Drawing for the job (mm, zero at the part's lowest x, y, z). A direction names the side the tool comes from. Round coordinates to 2 decimals unless told otherwise and drop trailing zeros. Write each loop counter-clockwise with the first axis right and the second up, starting at its lowest first coordinate (ties: lowest second). Pieces come first, ordered by that corner, then holes. Notation, with made-up numbers: M -1.75,-33.5 L 17.25,-33.5 A14 ccw 17.25,-14.5 Z; hole C 74.25,7.25 d2. An arc over 180 degrees is marked long. Use a Markdown table: item, result. Add a question column.
1) Wall check: probe 1 along Y at (x, z) = (31.75, 2.1); probe 2 along Z at (x, y) = (6, 2); probe 3 along Z at (x, y) = (31, 4.75). Give the ranges that are in metal, low to high.
2) Drop flat-ended pins along their axis: P1, Ø3, axis at x = 52.5, y = 2, coming from the +Z side; P2, Ø8.5, axis at x = 31.75, z = 9.525, coming from the +Y side; P3, Ø1, axis at y = 5, z = 14, coming from the -X side; P4, Ø1, axis at y = 4.5, z = 14, coming from the +X side. Give the stop position or say it passes through.
3) Slice it at D-D on x = 21.5. Write the cut outline in (y, z).
4) Two-plate mould, pull along Z, no slides. Class the marked faces 1, 2, 3 and 4: released by +Z, released by -Z, zero draft, split by the parting line, or undercut.
5) Slice it at C-C on z = 10.75. Write the cut outline in (x, y), plus the area to 3 significant figures.
6) Slice it at A-A on x = 31.75. Write the cut outline in (y, z).
7) Which spindle directions (+Z, -Z, +X, -X, +Y, -Y) get a long thin tool onto all of the face, cutting with end or side? Do the marked faces 5, 6 and 7. Say none if no direction does.
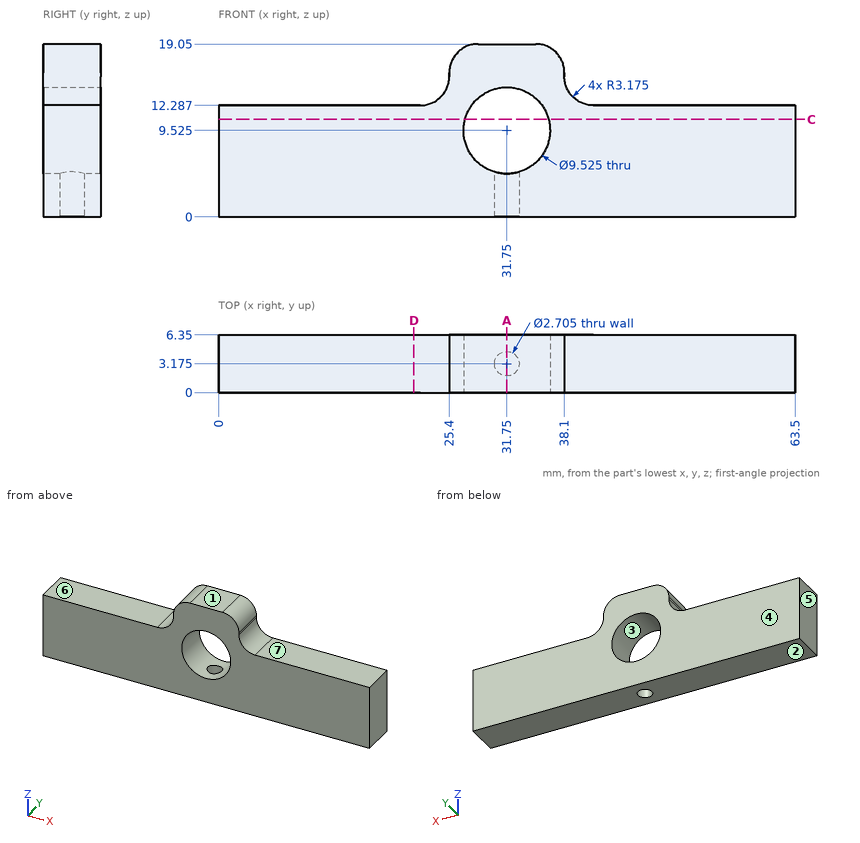
Entries:
| question | item | result |
|---|---|---|
| 1 | probe 1 | y = 0 to 1.82, 4.53 to 6.35 |
| 1 | probe 2 | z = 0 to 12.29 |
| 1 | probe 3 | z = 0 to 4.82, 14.23 to 19.05 |
| 2 | P1 | stops at z = 12.29 |
| 2 | P2 | passes through |
| 2 | P3 | stops at x = 24.72 |
| 2 | P4 | stops at x = 38.78 |
| 3 | outline | M 0,0 L 6.35,0 L 6.35,12.29 L 0,12.29 Z |
| 4 | face 1 | released by +Z |
| 4 | face 2 | released by -Z |
| 4 | face 3 | undercut |
| 4 | face 4 | zero draft |
| 5 | outline | M 0,0 L 27.15,0 L 27.15,6.35 L 0,6.35 Z; M 36.35,0 L 63.5,0 L 63.5,6.35 L 36.35,6.35 Z |
| 5 | area | 345 mm^2 |
| 6 | outline | M 0,0 L 1.82,0 L 1.82,4.76 L 0,4.76 Z; M 0,14.29 L 6.35,14.29 L 6.35,19.05 L 0,19.05 Z; M 4.53,0 L 6.35,0 L 6.35,4.76 L 4.53,4.76 Z |
| 7 | face 5 | +Z, -Z, -X, +Y, -Y |
| 7 | face 6 | +Z, -X, +Y, -Y |
| 7 | face 7 | +Z, +X, +Y, -Y |
